```python
from build123d import *

# Parameters (mm, degrees)
SKETCH1_R             = 2.5
SKETCH1_R_2           = 0.85
BOSS_EXTRUDE1_DEPTH   = 8
BOSS_EXTRUDE1_2_DEPTH = 8
SKETCH2_R             = 2.5
BOSS_EXTRUDE2_DEPTH   = 14.4
BOSS_EXTRUDE3_DEPTH   = 5
BOSS_EXTRUDE4_DEPTH   = 15.4


with BuildPart() as part:
    # Sketch1 → Boss-Extrude1 (new body)
    with BuildSketch(Plane(origin=(21.67087115, 151.425949174, 0), x_dir=(0.989914142, -0.141668597, 0), z_dir=(0.141668597, 0.989914142, 0))):
        with Locations((75.952188142, -57.025881449)):
            Circle(SKETCH1_R)
        with Locations((75.952188142, -57.025881449)):
            Circle(SKETCH1_R_2, mode=Mode.SUBTRACT)
    extrude(amount=BOSS_EXTRUDE1_DEPTH)



with BuildPart() as body_2:
    # Sketch1 → Boss-Extrude1 2 (new body)
    with BuildSketch(Plane(origin=(21.67087115, 151.425949174, 0), x_dir=(0.989914142, -0.141668597, 0), z_dir=(0.141668597, 0.989914142, 0))):
        with Locations((50.752188142, -57.025881449)):
            Circle(SKETCH1_R)
        with Locations((50.752188142, -57.025881449)):
            Circle(SKETCH1_R_2, mode=Mode.SUBTRACT)
    extrude(amount=BOSS_EXTRUDE1_2_DEPTH)


with BuildPart() as part_1:
    add(part.part)

    add(body_2.part)  # Boss-Extrude2 merges body 2
    # Sketch2 → Boss-Extrude2 (add)
    with BuildSketch(Plane(origin=(22.804219929, 159.34526231, 0), x_dir=(0.989914142, -0.141668597, 0), z_dir=(0.141668597, 0.989914142, 0))):
        with Locations((75.952188142, -57.025881449)):
            Circle(SKETCH2_R)
        with Locations((50.752188142, -57.025881449)):
            Circle(SKETCH2_R)
    extrude(amount=BOSS_EXTRUDE2_DEPTH)

    # Sketch3 → Boss-Extrude3 (add)
    with BuildSketch(Plane(origin=(24.84424773, 173.600025954, 0), x_dir=(0.989914142, -0.141668597, 0), z_dir=(0.141668597, 0.989914142, 0))):
        with BuildLine():
            ThreePointArc((53.252188142, -57.025881449), (53.984421189, -55.258114497), (55.752188142, -54.525881449))
            Line((55.752188142, -54.525881449), (70.952188142, -54.525881449))
            ThreePointArc((70.952188142, -54.525881449), (72.719955095, -55.258114497), (73.452188142, -57.025881449))
            ThreePointArc((73.452188142, -57.025881449), (75.952188142, -54.525881449), (78.452188142, -57.025881449))
            Line((78.452188142, -57.025881449), (78.452188142, -53.525881449))
            ThreePointArc((78.452188142, -53.525881449), (77.573508485, -51.404561106), (75.452188142, -50.525881449))
            Line((75.452188142, -50.525881449), (51.252188142, -50.525881449))
            ThreePointArc((51.252188142, -50.525881449), (49.130867798, -51.404561106), (48.252188142, -53.525881449))
            Line((48.252188142, -53.525881449), (48.252188142, -57.025881449))
            Line((48.252188142, -57.025881449), (53.252188142, -57.025881449))
        make_face()
    extrude(amount=-BOSS_EXTRUDE3_DEPTH)

    # Sketch4 → Boss-Extrude4 (add)
    with BuildSketch(Plane(origin=(24.135904744, 168.650455244, 0), x_dir=(0.989914142, -0.141668597, 0), z_dir=(-0.141668597, -0.989914142, 0))):
        with BuildLine():
            Line((53.252188142, 57.025881449), (53.252188142, 52.525881449))
            ThreePointArc((53.252188142, 52.525881449), (52.666401704, 51.111667887), (51.252188142, 50.525881449))
            ThreePointArc((51.252188142, 50.525881449), (49.130867798, 51.404561106), (48.252188142, 53.525881449))
            Line((48.252188142, 53.525881449), (48.252188142, 57.025881449))
            ThreePointArc((48.252188142, 57.025881449), (50.752188142, 54.525881449), (53.252188142, 57.025881449))
        make_face()
        with BuildLine():
            Line((73.452188142, 57.025881449), (73.452188142, 52.525881449))
            ThreePointArc((73.452188142, 52.525881449), (74.037974579, 51.111667887), (75.452188142, 50.525881449))
            ThreePointArc((75.452188142, 50.525881449), (77.573508485, 51.404561106), (78.452188142, 53.525881449))
            Line((78.452188142, 53.525881449), (78.452188142, 57.025881449))
            ThreePointArc((78.452188142, 57.025881449), (75.952188142, 54.525881449), (73.452188142, 57.025881449))
        make_face()
    extrude(amount=BOSS_EXTRUDE4_DEPTH)

    # Sketch9 → Cut-Loft7 section 0
    with BuildSketch(Plane(origin=(21.954208345, 153.405777458, 0), x_dir=(0.989914142, -0.141668597, 0), z_dir=(-0.141668597, -0.989914142, 0))):
        with BuildLine():
            Line((48.252188142, 57.025881449), (43.252188142, 57.025881449))
            ThreePointArc((43.252188142, 57.025881449), (45.448887283, 51.722580591), (50.752188142, 49.525881449))
            ThreePointArc((50.752188142, 49.525881449), (56.055489001, 51.722580591), (58.252188142, 57.025881449))
            Line((58.252188142, 57.025881449), (53.252188142, 57.025881449))
            ThreePointArc((53.252188142, 57.025881449), (52.519955095, 55.258114497), (50.752188142, 54.525881449))
            ThreePointArc((50.752188142, 54.525881449), (48.984421189, 55.258114497), (48.252188142, 57.025881449))
        make_face()
    # Sketch8 → Cut-Loft7 section 1
    with BuildSketch(Plane(origin=(24.135904744, 168.650455244, 0), x_dir=(0.989914142, -0.141668597, 0), z_dir=(-0.141668597, -0.989914142, 0))):
        with BuildLine():
            Line((48.252188142, 53.525881449), (45.252188142, 53.525881449))
            ThreePointArc((45.252188142, 53.525881449), (47.009547455, 49.283240762), (51.252188142, 47.525881449))
            ThreePointArc((51.252188142, 47.525881449), (54.787722048, 48.990347544), (56.252188142, 52.525881449))
            Line((56.252188142, 52.525881449), (53.252188142, 52.525881449))
            ThreePointArc((53.252188142, 52.525881449), (52.666401704, 51.111667887), (51.252188142, 50.525881449))
            ThreePointArc((51.252188142, 50.525881449), (49.130867798, 51.404561106), (48.252188142, 53.525881449))
        make_face()
    loft(mode=Mode.SUBTRACT)

    # Sketch9<3> → Cut-Loft8 section 0
    with BuildSketch(Plane(origin=(21.954208345, 153.405777458, 0), x_dir=(0.989914142, -0.141668597, 0), z_dir=(-0.141668597, -0.989914142, 0))):
        with BuildLine():
            Line((73.452188142, 57.025881449), (68.452188142, 57.025881449))
            ThreePointArc((68.452188142, 57.025881449), (70.648887283, 51.722580591), (75.952188142, 49.525881449))
            ThreePointArc((75.952188142, 49.525881449), (81.255489001, 51.722580591), (83.452188142, 57.025881449))
            Line((83.452188142, 57.025881449), (78.452188142, 57.025881449))
            ThreePointArc((78.452188142, 57.025881449), (77.719955095, 55.258114497), (75.952188142, 54.525881449))
            ThreePointArc((75.952188142, 54.525881449), (74.184421189, 55.258114497), (73.452188142, 57.025881449))
        make_face()
    # Sketch8<8> → Cut-Loft8 section 1
    with BuildSketch(Plane(origin=(24.135904744, 168.650455244, 0), x_dir=(0.989914142, -0.141668597, 0), z_dir=(-0.141668597, -0.989914142, 0))):
        with BuildLine():
            Line((73.452188142, 52.525881449), (70.452188142, 52.525881449))
            ThreePointArc((70.452188142, 52.525881449), (71.916654236, 48.990347544), (75.452188142, 47.525881449))
            ThreePointArc((75.452188142, 47.525881449), (79.694828829, 49.283240762), (81.452188142, 53.525881449))
            Line((81.452188142, 53.525881449), (78.452188142, 53.525881449))
            ThreePointArc((78.452188142, 53.525881449), (77.573508485, 51.404561106), (75.452188142, 50.525881449))
            ThreePointArc((75.452188142, 50.525881449), (74.037974579, 51.111667887), (73.452188142, 52.525881449))
        make_face()
    loft(mode=Mode.SUBTRACT)


solid = part_1.part
```
For this review, take the finished solid that the model builds, in its own axes (mm). A direction names the side the tool comes from. Round coordinates to 2 decimals unless told otherwise and drop trailing zeros. Order: outer loops, then holes, each group sorted by start corner. A loop starts at its lowest first (then second) coordinate and runs counter-clockwise, first axis right, second up. Notation, with made-up numbers: (83, 79) -> (139, 79) arc R19 cw to (139, 105) -> close; hole circle Ø3 at (15, 79.5). An arc over 180 degrees is marked (long way). Use a Markdown table: item, result.
Item 1: Take a section at D-D (x = 82). State the section outline as (y, z) points.
Resolved:
| item | result |
|---|---|
| outline | (160.37, 50.53) -> (165.42, 50.53) -> (165.42, 54.53) -> (160.37, 54.53) -> close |
Item 2: For line 1 along X through (y, z) = (150, 57); line 2 along X through (y, z) = (147.75, 54.5); line 3 along X through (y, z) = (156.5, 56.25), list the stretches that pass through material, from the lowest coordinate up. Write a range as [from, to].
Resolved:
| item | result |
|---|---|
| line 1 | x = [70.21, 71.88], [73.59, 75.26], [95.67, 100.72] |
| line 2 | x = [71.19, 73.87], [95.63, 100.07] |
| line 3 | x = [71.14, 76.19], [96.6, 101.65] |
Item 3: Machinability: for faces 4 (the flat face through (87, 162, 50.526)), 5 (the flat face through (73.033, 152.157, 57.014)), 6 (the flat face through (96.014, 152.423, 55.307)), 7 (the flat face through (76.018, 155.285, 55.307)), which of the approach directions +Z, -Z, +X, -X, +Y, -Y give a long, thin tool a straight path to every point of the face, cutting with its end or side? Answer none if there is none.
Resolved:
| item | result |
|---|---|
| face 4 | -Z, +X, -X, +Y, -Y |
| face 5 | none |
| face 6 | +Z, -Z |
| face 7 | +Z, -Z, -Y |
Item 4: Take a section at A-A (z = 58.75). State the section outline as (x, y) points.
Resolved:
| item | result |
|---|---|
| outline | (70.12, 144.49) -> (73.7, 143.98) -> (76.88, 166.15) -> (73.29, 166.67) -> close; (95.06, 140.92) -> (98.65, 140.41) -> (101.82, 162.58) -> (98.24, 163.1) -> close |
Item 5: Draft analysis for pull direction Z (two halves, no side actions). For faces 1 (the flat face through (87, 162, 54.526)), 2 (the flat face through (97.979, 148.587, 57.014)), 3 (the flat face through (71.88, 144.24, 58.1)), state which applies: +Z half, -Z half, draft (parallel to the pull), parting line (faces both ways), or undercut.
Resolved:
| item | result |
|---|---|
| face 1 | +Z half |
| face 2 | undercut |
| face 3 | draft |
Item 6: For pin 1 (1.5 mm diameter, centred on y = 157.5, z = 57, fed in from +X); pin 2 (2 mm diameter, centred on y = 155, z = 54.5, fed in from +X); pin 3 (4 mm diameter, centred on y = 149.5, z = 52, fed in from +X); pin 4 (6 mm diameter, centred on x = 98.5, y = 144.5, fed in from +Z), all flat-tipped, find the tip position at first contact; note any pin that passes through.
Resolved:
| item | result |
|---|---|
| pin 1 | stops at x = 101.9 |
| pin 2 | stops at x = 101.58 |
| pin 3 | stops at x = 100.4 |
| pin 4 | stops at z = 59.53 |
Item 7: Take a section at B-B (y = 151.25). State how many separate pieces and enclosed holes the cut face has, plus the area to 3 significant figures.
Resolved:
| item | result |
|---|---|
| separate pieces | 2 |
| enclosed holes | 1 |
| area | 55.4 mm² |
